CAD build for the part. Positions are in the model's coordinates, mm. Face numbers are marked on the shaded views. A direction names the side the tool comes from. Round coordinates to 2 decimals unless told otherwise and drop trailing zeros. Loops run counter-clockwise (first coordinate to the right, second up) from the corner with the lowest first, then second, coordinate; pieces in that order, holes last.
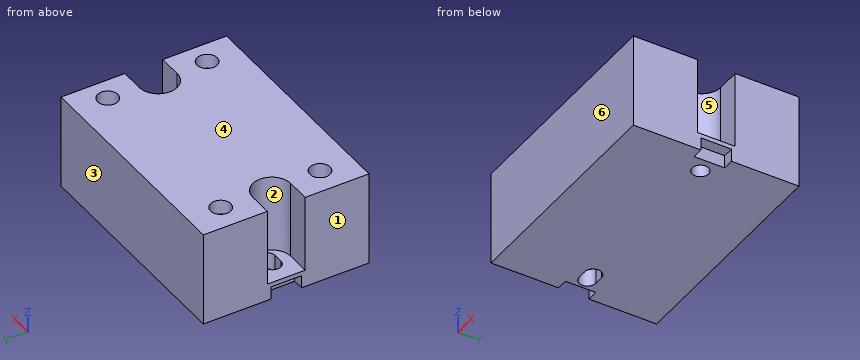
from build123d import *

# Parameters (mm, degrees)
F0_W     = 62.7
F0_H     = 45
F1_DEPTH = 25.7
F3_DEPTH = 3.5
F5_DEPTH = 21
F6_R     = 2.25
F7_DEPTH = 4.7
F9_D     = 5.5
F9_DEPTH = 4
F9_TIP   = 1.6523667023


with BuildPart() as f1:
    # F0 (on Top) → F1 (new body)
    with BuildSketch(Plane.XY):
        with Locations((31.35, 22.5)):
            Rectangle(F0_W, F0_H)
    extrude(amount=F1_DEPTH)

    # F2 (on face) → F3 (cut)
    with BuildSketch(Plane(origin=(0, 0, 0), x_dir=(1, 0, 0), z_dir=(0, 0, -1))):
        Polygon((0, -18.35), (0, -22.5), (0, -26.65), (3, -26.65), (3, -22.5), (3, -18.35), align=None)
        Polygon((62.7, -22.5), (62.7, -18.35), (59.7, -18.35), (59.7, -22.5), (59.7, -26.65), (62.7, -26.65), align=None)
    extrude(amount=-F3_DEPTH, mode=Mode.SUBTRACT)

    # F4 (on face) → F5 (cut)
    with BuildSketch(Plane.XY.offset(25.7)):
        with BuildLine():
            Line((0, 27.65), (0, 22.5))
            Line((0, 22.5), (0, 17.35))
            Line((0, 17.35), (6.35, 17.35))
            ThreePointArc((6.35, 17.35), (11.5, 22.5), (6.35, 27.65))
            Line((6.35, 27.65), (0, 27.65))
        make_face()
        with BuildLine():
            ThreePointArc((56.35, 27.65), (51.2, 22.5), (56.35, 17.35))
            Line((56.35, 17.35), (62.7, 17.35))
            Line((62.7, 17.35), (62.7, 22.5))
            Line((62.7, 22.5), (62.7, 27.65))
            Line((62.7, 27.65), (56.35, 27.65))
        make_face()
    extrude(amount=-F5_DEPTH, mode=Mode.SUBTRACT)

    # F6 (on face) → F7 (cut, through all)
    with BuildSketch(Plane(origin=(0, 0, 0), x_dir=(1, 0, 0), z_dir=(0, 0, -1))):
        with Locations((55.75, -22.5)):
            Circle(F6_R)
        with BuildLine():
            Line((8.4999779246, -20.2500000001), (6.0104839369, -20.2500244252))
            ThreePointArc((6.0104839369, -20.2500244252), (3.750330021, -22.5385355083), (6.087536662, -24.7482965402))
            Line((6.087536662, -24.7482965402), (8.4984107338, -24.7499994387))
            ThreePointArc((8.4984107338, -24.7499994387), (10.7499998636, -22.5007835955), (8.4999779246, -20.2500000001))
        make_face()
    extrude(amount=-F7_DEPTH, mode=Mode.SUBTRACT)

    # F9
    with Locations(Plane.XY.offset(25.7)):
        with Locations((7, 36), (7, 9), (56.7, 9), (56.7, 36)):
            Hole(F9_D / 2, depth=F9_DEPTH)
            with Locations((0, 0, -(F9_DEPTH + F9_TIP / 2))):  # 118° drill point
                Cone(0, F9_D / 2, F9_TIP, mode=Mode.SUBTRACT)


solid = f1.part
Item 1: Cut at A-A (z = 13.5). List the corners of the cut face in (x, y), plus the area to 3 significant figures.
Verdict:
outline: (0, 0) - (62.7, 0) - (62.7, 17.35) - (56.35, 17.35) arc R5.15 cw to (56.35, 27.65) - (62.7, 27.65) - (62.7, 45) - (0, 45) - (0, 27.65) - (6.35, 27.65) arc R5.15 cw to (6.35, 17.35) - (0, 17.35) - close
area: 2,610 mm2
Item 2: Wall check: L1, parallel to X at y = 9, z = 22.55; L2, parallel to Y at x = 56.7, z = 23.45; L3, parallel to X at y = 22.5, z = 1.45. Give the ranges that are in metal, low to high.
Verdict:
L1: x = 0 to 4.25, 9.75 to 53.95, 59.45 to 62.7
L2: y = 0 to 6.25, 11.75 to 17.35, 27.65 to 33.25, 38.75 to 45
L3: x = 3 to 3.75, 10.75 to 53.5, 58 to 59.7
Item 3: Flat gauge pins, fed straight in: P1, Ø1.5, axis at x = 2, y = 23, coming from the -Z side; P2, Ø0.9, axis at x = 60.5, z = 2, coming from the -Y side; P3, Ø5, axis at x = 7, y = 36, coming from the +Z side. Where does each tip first touch, or does it go through?
Verdict:
P1: stops at z = 3.5
P2: stops at y = 0
P3: stops at z = 21.55
Item 4: Mould opens along Y. For the marked faces 3, 4, 5 and 6 say: released by +Y, released by -Y, zero draft, split by the parting line, or undercut.
Verdict:
face 3: released by +Y
face 4: zero draft
face 5: undercut
face 6: released by -Y
Item 5: 3-axis set-ups, long thin cutter, end or side, ignore diameter. For the marked faces 1 and 2: which of +Z, -Z, +X, -X, +Y, -Y reach the whole face in a straight line?
Verdict:
face 1: +Z, -Z, -X, +Y, -Y
face 2: +Z, -X
